The figure shows three views and two pictorial views of one solid part (mm, origin at its lowest corner). Answer the questions. A direction names the side the tool comes from. Round coordinates to 2 decimals unless told otherwise and drop trailing zeros. Order: outer loops, then holes, each group sorted by start corner. A loop starts at its lowest first (then second) coordinate and runs counter-clockwise, first axis right, second up. Notation, with made-up numbers: (-32.75, -33.5) - (19.25, -33.5) arc R22 cw to (19.25, -24.5) - close; hole circle Ø10 at (63.5, -10.5). An arc over 180 degrees is marked (long way). Answer in a Markdown table with one row per item.
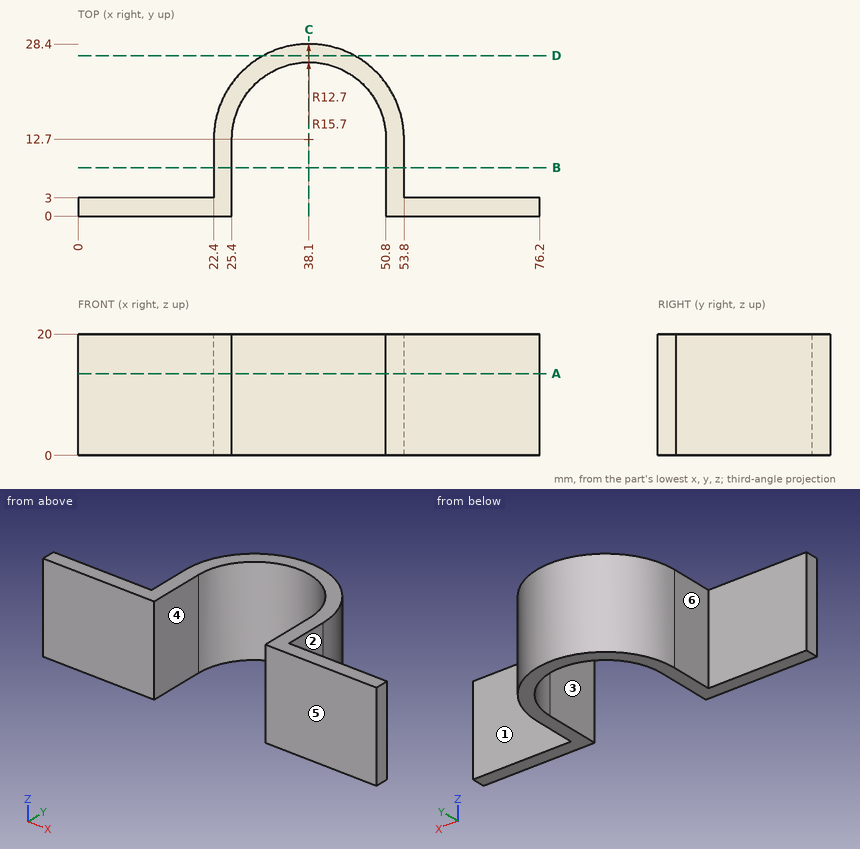
1) Find section D-D, the plane y = 26.5. Give the vertices of the cut face in (x, z), then the cut area to 3 significant figures.
Filled in:
| item | result |
|---|---|
| outline | (30.61, 0) - (45.59, 0) - (45.59, 20) - (30.61, 20) - close |
| area | 299 mm^2 |
2) Find section C-C, the plane x = 38.1. Give the vertices of the cut face in (y, z), then the cut area to 3 significant figures.
Filled in:
| item | result |
|---|---|
| outline | (25.4, 0) - (28.4, 0) - (28.4, 20) - (25.4, 20) - close |
| area | 60.0 mm^2 |
3) Find section A-A, the plane z = 13.5. Give the vertices of the cut face in (x, y), then the cut area to 3 significant figures.
Filled in:
| item | result |
|---|---|
| outline | (0, 0) - (25.4, 0) - (25.4, 12.7) arc R12.7 cw to (50.8, 12.7) - (50.8, 0) - (76.2, 0) - (76.2, 3) - (53.8, 3) - (53.8, 12.7) arc R15.7 ccw to (22.4, 12.7) - (22.4, 3) - (0, 3) - close |
| area | 344 mm^2 |
4) Find section B-B, the plane y = 8. Give the vertices of the cut face in (x, z).
Filled in:
| item | result |
|---|---|
| outline | (22.4, 0) - (25.4, 0) - (25.4, 20) - (22.4, 20) - close; (50.8, 0) - (53.8, 0) - (53.8, 20) - (50.8, 20) - close |
5) Find the intervals of material crossed by probe 1 along X at (y, z) = (7.75, 11.5); probe 2 along X at (y, z) = (2.25, 18); probe 3 along Y at (x, z) = (57, 12), in increasing order. Write a range as from..to.
Filled in:
| item | result |
|---|---|
| probe 1 | x = 22.4..25.4, 50.8..53.8 |
| probe 2 | x = 0..25.4, 50.8..76.2 |
| probe 3 | y = 0..3 |
6) Which of the six approach directions +Z, -Z, +X, -X, +Y, -Y give full straight-line access (tool end or side, diameter ignored) to the marked faces 4, 5 and 6?
Filled in:
| item | result |
|---|---|
| face 4 | +Z, -Z, -Y |
| face 5 | +Z, -Z, +X, -X, -Y |
| face 6 | +Z, -Z, -X, +Y |
7) Each of these flat-tipped pins is pushed along its axis until it touches: pin 1 (3 mm diameter, centred on y = 5.5, z = 12, fed in from +X); pin 2 (2 mm diameter, centred on x = 53, z = 6, fed in from +Y); pin 3 (8 mm diameter, centred on y = 12.5, z = 6, fed in from -X). Where does it stop, or does it pass through?
Filled in:
| item | result |
|---|---|
| pin 1 | stops at x = 53.8 |
| pin 2 | stops at y = 20 |
| pin 3 | stops at x = 22.4 |
8) The mould has two halves that part along X. Classify the marked faces 1, 2 and 3: released by +X, released by -X, zero draft, split by the parting line, or undercut.
Filled in:
| item | result |
|---|---|
| face 1 | zero draft |
| face 2 | released by +X |
| face 3 | undercut |
